CAD build for the part. Positions are in the model's coordinates, mm. Face numbers are marked on the shaded views. Coordinates: 2 decimals unless noted, no trailing zeros. Loops run counter-clockwise (first coordinate to the right, second up) from the corner with the lowest first, then second, coordinate; pieces in that order, holes last.
1) Pin check, flat tips, straight feed: pin 1 Ø0.8 at (x, y) = (49.5, 0.5) entering from +Z; pin 2 Ø6 at (x, y) = (24, 11) entering from +Z; pin 3 Ø1.4 at (y, z) = (1, -49) entering from -X; pin 4 Ø4 at (x, z) = (-24.7, -46.8) entering from -Y. Stop position of each tip, or through.
2) Saw through at A-A, the plane x = -17.5. Write the cut outline in (y, z).
3) Saw through at D-D, the plane x = 45.2. Write the cut outline in (y, z).
4) Two-plate mould, pull along Z, no slides. Class the marked faces 1 and 2: +Z half, -Z half, draft (parallel to the pull), parting line (faces both ways), or undercut.
5) Saw through at C-C, the plane y = 11. Write the cut outline in (x, z), and give its area (3 significant figures).
6) Wall check: line 1 along X through (y, z) = (6.8, -30) (3 decimals); line 2 along Z through (x, y) = (-45.2, 0.8). Give the ranges that are in metal, low to high.
7) Saw through at B-B, the plane z = -9.5. Write the cut outline in (x, y), and give its area (3 significant figures).
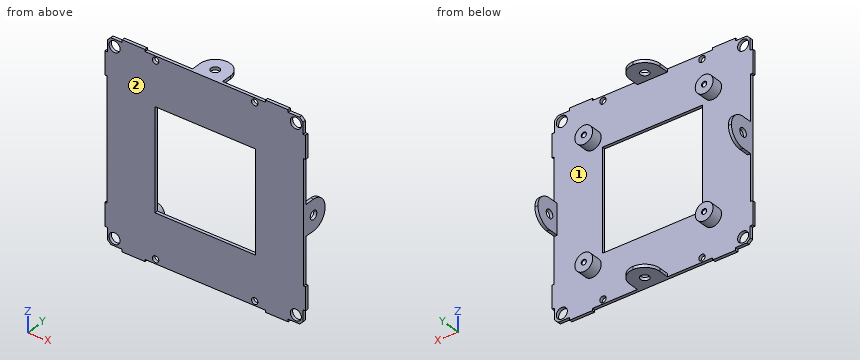
```python
from build123d import *

# Parameters (mm, degrees)
SKETCH1_R                 = 2.7503
SKETCH1_R_2               = 1.575
SKETCH1_W                 = 50
SKETCH1_H                 = 50
BOSS_EXTRUDE1_DEPTH       = 1.524
SKETCH2_W                 = 15
SKETCH2_H                 = 2.5
SKETCH2_W_2               = 2.5
SKETCH2_H_2               = 15
BOSS_EXTRUDE2_DEPTH       = 12.476
SKETCH3_R                 = 2.125
CUT_EXTRUDE1_DEPTH        = 1
CUT_EXTRUDE1_DEPTH_BACK   = 101
SKETCH4_R                 = 2.125
CUT_EXTRUDE2_DEPTH        = 1
CUT_EXTRUDE2_DEPTH_BACK   = 101
SKETCH5_W                 = 60
SKETCH5_H                 = 1
SKETCH5_W_2               = 1
SKETCH5_H_2               = 60
CUT_EXTRUDE3_DEPTH        = 1
CUT_EXTRUDE3_DEPTH_BACK   = 15
SKETCH6_R                 = 4.445
BOSS_EXTRUDE3_DEPTH       = 5.5
F_5_40_TAPPED_HOLE1_D     = 2.5781
F_5_40_TAPPED_HOLE1_DEPTH = 0.55
F_5_40_TAPPED_HOLE1_TIP   = 0.774539381


with BuildPart() as part:
    # Sketch1 → Boss-Extrude1 (new body)
    with BuildSketch(Plane(origin=(0, 0, 0), x_dir=(1, 0, 0), z_dir=(0, 1, 0))):
        Polygon((41.364, 50), (-41.364, 50), (-41.364, 48.73), (-47.079, 48.73), (-48.73, 47.079), (-48.73, 41.364), (-50, 41.364), (-50, -41.364), (-48.73, -41.364), (-48.73, -47.079), (-47.079, -48.73), (-41.364, -48.73), (-41.364, -50), (41.364, -50), (41.364, -48.73), (47.079, -48.73), (48.73, -47.079), (48.73, -41.364), (50, -41.364), (50, 41.364), (48.73, 41.364), (48.73, 47.079), (47.079, 48.73), (41.364, 48.73), align=None)
        with Locations((-45.2, -45.2)):
            Circle(SKETCH1_R, mode=Mode.SUBTRACT)
        with Locations((-24.7, -46.8)):
            Circle(SKETCH1_R_2, mode=Mode.SUBTRACT)
        with Locations((24.7, -46.8)):
            Circle(SKETCH1_R_2, mode=Mode.SUBTRACT)
        with Locations((45.2, -45.2)):
            Circle(SKETCH1_R, mode=Mode.SUBTRACT)
        Rectangle(SKETCH1_W, SKETCH1_H, mode=Mode.SUBTRACT)
        with Locations((-45.2, 45.2)):
            Circle(SKETCH1_R, mode=Mode.SUBTRACT)
        with Locations((-24.7, 46.8)):
            Circle(SKETCH1_R_2, mode=Mode.SUBTRACT)
        with BuildLine():
            ThreePointArc((26.275, 46.8), (24.7, 45.225), (23.125, 46.8))
            ThreePointArc((23.125, 46.8), (24.7, 48.375), (26.275, 46.8))
        make_face(mode=Mode.SUBTRACT)
        with Locations((45.2, 45.2)):
            Circle(SKETCH1_R, mode=Mode.SUBTRACT)
    extrude(amount=BOSS_EXTRUDE1_DEPTH)

    # Sketch2 → Boss-Extrude2 (add)
    with BuildSketch(Plane(origin=(0, 1.524, 0), x_dir=(1, 0, 0), z_dir=(0, 1, 0))):
        with Locations((0, 48.75)):
            Rectangle(SKETCH2_W, SKETCH2_H)
        with Locations((48.75, 0)):
            Rectangle(SKETCH2_W_2, SKETCH2_H_2)
        with Locations((0, -48.75)):
            Rectangle(SKETCH2_W, SKETCH2_H)
        with Locations((-48.75, 0)):
            Rectangle(SKETCH2_W_2, SKETCH2_H_2)
    extrude(amount=BOSS_EXTRUDE2_DEPTH)

    # Sketch3 → Cut-Extrude1 (cut, two sides)
    with BuildSketch(Plane.XY.offset(50)) as cut_extrude1_sk:
        with BuildLine():
            ThreePointArc((0, 14), (5.303300859, 11.803300859), (7.5, 6.5))
            Line((7.5, 6.5), (7.5, 14))
            Line((7.5, 14), (0, 14))
        make_face()
        with BuildLine():
            ThreePointArc((-7.5, 6.5), (-5.303300859, 11.803300859), (0, 14))
            Line((0, 14), (-7.5, 14))
            Line((-7.5, 14), (-7.5, 6.5))
        make_face()
        with Locations((0, 6.5)):
            Circle(SKETCH3_R)
    extrude(amount=CUT_EXTRUDE1_DEPTH, mode=Mode.SUBTRACT)
    extrude(cut_extrude1_sk.sketch, amount=-CUT_EXTRUDE1_DEPTH_BACK, mode=Mode.SUBTRACT)

    # Sketch4 → Cut-Extrude2 (cut, two sides)
    with BuildSketch(Plane.ZY.offset(50)) as cut_extrude2_sk:
        with Locations((0, 6.5)):
            Circle(SKETCH4_R)
        with BuildLine():
            ThreePointArc((0, 14), (5.303300859, 11.803300859), (7.5, 6.5))
            Line((7.5, 6.5), (7.5, 14))
            Line((7.5, 14), (0, 14))
        make_face()
        with BuildLine():
            ThreePointArc((-7.5, 6.5), (-5.303300859, 11.803300859), (0, 14))
            Line((0, 14), (-7.5, 14))
            Line((-7.5, 14), (-7.5, 6.5))
        make_face()
    extrude(amount=CUT_EXTRUDE2_DEPTH, mode=Mode.SUBTRACT)
    extrude(cut_extrude2_sk.sketch, amount=-CUT_EXTRUDE2_DEPTH_BACK, mode=Mode.SUBTRACT)

    # Sketch5 → Cut-Extrude3 (cut, two sides)
    with BuildSketch(Plane.XZ) as cut_extrude3_sk:
        with Locations((0, -49.5)):
            Rectangle(SKETCH5_W, SKETCH5_H)
        with Locations((-49.5, 0)):
            Rectangle(SKETCH5_W_2, SKETCH5_H_2)
        with Locations((0, 49.5)):
            Rectangle(SKETCH5_W, SKETCH5_H)
        with Locations((49.5, 0)):
            Rectangle(SKETCH5_W_2, SKETCH5_H_2)
    extrude(amount=CUT_EXTRUDE3_DEPTH, mode=Mode.SUBTRACT)
    extrude(cut_extrude3_sk.sketch, amount=-CUT_EXTRUDE3_DEPTH_BACK, mode=Mode.SUBTRACT)

    # Sketch6 → Boss-Extrude3 (add)
    with BuildSketch(Plane(origin=(0, 1.524, 0), x_dir=(1, 0, 0), z_dir=(0, 1, 0))):
        with Locations((30, 30)):
            Circle(SKETCH6_R)
        with Locations((30, -30)):
            Circle(SKETCH6_R)
        with Locations((-30, -30)):
            Circle(SKETCH6_R)
        with Locations((-30, 30)):
            Circle(SKETCH6_R)
    extrude(amount=BOSS_EXTRUDE3_DEPTH)

    # #5-40 Tapped Hole1
    with Locations(Plane(origin=(0, 7.024, 0), x_dir=(1, 0, 0), z_dir=(0, 1, 0))):
        with Locations((-17.222965343, 16.834933913), (-30, 30), (-30, -30), (30, -30), (30, 30)):
            Hole(F_5_40_TAPPED_HOLE1_D / 2, depth=F_5_40_TAPPED_HOLE1_DEPTH)
            with Locations((0, 0, -(F_5_40_TAPPED_HOLE1_DEPTH + F_5_40_TAPPED_HOLE1_TIP / 2))):  # 118° drill point
                Cone(0, F_5_40_TAPPED_HOLE1_D / 2, F_5_40_TAPPED_HOLE1_TIP, mode=Mode.SUBTRACT)


solid = part.part
```
Data:
1. pin 1: stops at z = 41.36
1. pin 2: passes through
1. pin 3: stops at x = -47.51
1. pin 4: stops at y = 0
2. outline: (0, -49) - (1.52, -49) - (1.52, -25) - (0, -25) - close; (0, 25) - (1.52, 25) - (1.52, 49) - (0, 49) - close
3. outline: (0, -48.73) - (1.52, -48.73) - (1.52, -47.95) - (0, -47.95) - close; (0, -42.45) - (1.52, -42.45) - (1.52, 42.45) - (0, 42.45) - close; (0, 47.95) - (1.52, 47.95) - (1.52, 48.73) - (0, 48.73) - close
4. face 1: undercut
4. face 2: draft
5. outline: (-49, -6) - (-47.5, -6) - (-47.5, 6) - (-49, 6) - close; (-6, -49) - (6, -49) - (6, -47.5) - (-6, -47.5) - close; (-6, 47.5) - (6, 47.5) - (6, 49) - (-6, 49) - close; (47.5, -6) - (49, -6) - (49, 6) - (47.5, 6) - close
5. area: 72.0 mm2
6. line 1: x = -34.445 to -31.289, -28.711 to -25.555, 25.555 to 28.711, 31.289 to 34.445
6. line 2: z = -48.73 to -47.95, -42.45 to 42.45, 47.95 to 48.73
7. outline: (-49, 0) - (-25, 0) - (-25, 1.52) - (-49, 1.52) - close; (25, 0) - (49, 0) - (49, 1.52) - (25, 1.52) - close
7. area: 73.2 mm2
